The figure shows three views and two pictorial views of one solid part (mm, origin at its lowest corner). Answer the questions. A direction names the side the tool comes from. Round coordinates to 2 decimals unless told otherwise and drop trailing zeros. Loops run counter-clockwise (first coordinate to the right, second up) from the corner with the lowest first, then second, coordinate; pieces in that order, holes last. Notation, with made-up numbers: (-10, -5) - (30, -5) arc R21 cw to (30, 31) - close; hole circle Ø11 at (89.25, 40). An arc over 180 degrees is marked (long way). Use one line per item in the form item = value. Start each with the question number.
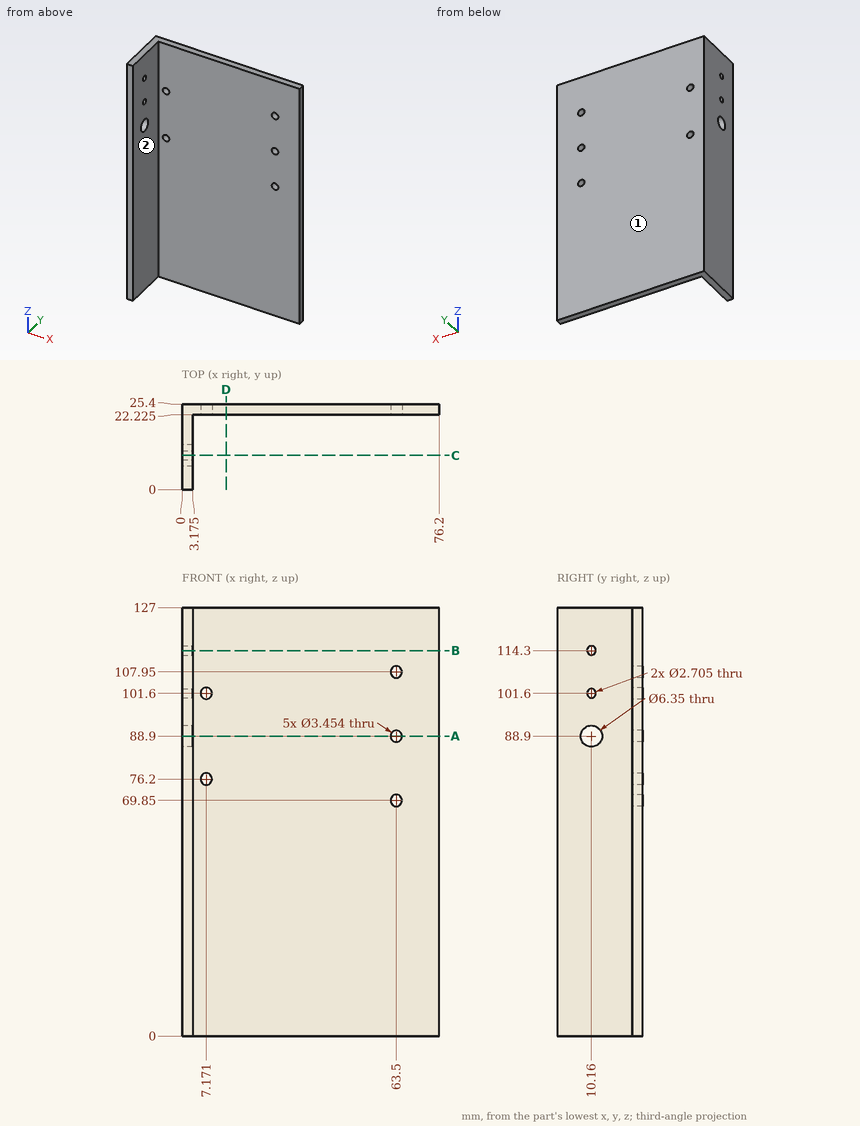
1) A cutting plane is placed at A-A on z = 88.9. Write down the section's boundary in (x, y) (1 decimal).
2) A cutting plane is placed at C-C on y = 10.16. Write down the section's boundary in (x, z) (1 decimal), plus the area to 3 significant figures.
3) For the marked faces 1 and 2, determine the directions among +Z, -Z, +X, -X, +Y, -Y from which every point of the face is accessible in a straight line to the end or side of a thin tool.
4) A cutting plane is placed at B-B on z = 114.3. Write down the section's boundary in (x, y) (1 decimal).
5) A cutting plane is placed at D-D on x = 13. Write down the section's boundary in (y, z) (1 decimal), plus the area to 3 significant figures.
6) Straight lines are drawn through the part: line 1 (Z direction, x = 63.5, y = 24.6); line 2 (Y direction, x = 1.55, z = 88.9) (1 decimal); line 3 (X direction, y = 24.7, z = 69.85). For each, find the intervals that lie inside material, in ascending order. Write a range as from..to.
7) Flat-ended cylindrical pins translate along their axes: pin 1 (2 mm diameter, centred on x = 15, z = 71.5, fed in from -Y) (1 decimal); pin 2 (1.5 mm diameter, centred on y = 11.5, z = 99, fed in from +X) (1 decimal); pin 3 (2 mm diameter, centred on x = 63.5, z = 88.9, fed in from +Y). Find the tip coordinate at first contact, or state that the pin passes through.
Checks:
q1.outline = (0, 0) - (3.2, 0) - (3.2, 7) - (0, 7) - close; (0, 13.3) - (3.2, 13.3) - (3.2, 22.2) - (61.8, 22.2) - (61.8, 25.4) - (0, 25.4) - close; (65.2, 22.2) - (76.2, 22.2) - (76.2, 25.4) - (65.2, 25.4) - close
q2.outline = (0, 0) - (3.2, 0) - (3.2, 85.7) - (0, 85.7) - close; (0, 92.1) - (3.2, 92.1) - (3.2, 100.2) - (0, 100.2) - close; (0, 103) - (3.2, 103) - (3.2, 112.9) - (0, 112.9) - close; (0, 115.7) - (3.2, 115.7) - (3.2, 127) - (0, 127) - close
q2.area = 366 mm²
q3.face_1 = +Z, -Z, +X, -X, +Y
q3.face_2 = +Z, -Z, +X, -Y
q4.outline = (0, 0) - (3.2, 0) - (3.2, 8.8) - (0, 8.8) - close; (0, 11.5) - (3.2, 11.5) - (3.2, 22.2) - (76.2, 22.2) - (76.2, 25.4) - (0, 25.4) - close
q5.outline = (22.2, 0) - (25.4, 0) - (25.4, 127) - (22.2, 127) - close
q5.area = 403 mm²
q6.line_1 = 0..68.12, 71.58..87.17, 90.63..106.22, 109.68..127
q6.line_2 = 0..7, 13.3..25.4
q6.line_3 = 0..61.77, 65.23..76.2
q7.pin_1 = 22.2
q7.pin_2 = 3.2
q7.pin_3 = through
